```python
from build123d import *


with BuildPart() as part:
    # Sketch1 → Body (revolve)
    with BuildSketch(Plane.XY):
        with BuildLine():
            Line((0, 21), (5, 21))
            Line((5, 21), (5, 18))
            Line((5, 18), (9, 18))
            Line((9, 18), (9, 21.75))
            Line((9, 21.75), (15.9, 21.75))
            ThreePointArc((15.9, 21.75), (20.001219331, 23.448780669), (21.7, 27.55))
            Line((21.7, 27.55), (21.7, 40.25))
            Line((21.7, 40.25), (25.3, 40.25))
            Line((25.3, 40.25), (25.3, 61))
            Line((25.3, 61), (5, 61))
            Line((5, 61), (5, 66))
            Line((5, 66), (0, 66))
            Line((0, 66), (0, 21))
        make_face()
    revolve(axis=Axis((0, 0, 0), (1, 0, 0)))


solid = part.part
```
Model file for the job. Use its own axes, mm. A direction names the side the tool comes from. Coordinates: 2 decimals unless noted, no trailing zeros. Write each loop counter-clockwise with the first axis right and the second up, starting at its lowest first coordinate (ties: lowest second). Pieces come first, ordered by that corner, then holes. Notation, with made-up numbers: (-26, 67) - (20, 67) arc R9 ccw to (20, 81) - close; hole circle Ø8 at (2, 38.5). An arc over 180 degrees is marked (long way). One line per item, written item: value. Start each with the question number.
1. Tool access for faces 1 (the cylindrical face through (7.028, -2.343, 17.847)), 2 (the cylindrical face through (23.53, -40.21, 1.77)), 3 (the flat face through (5, -9, 16)): list every direction of +Z, -Z, +X, -X, +Y, -Y with a clear straight run to the whole face (end or side of a thin tool).
2. Slice it at C-C (y = 49). Write the cut outline in (x, z), plus the area to 3 significant figures.
3. Flat gauge pins, fed straight in: pin 1 (12 mm diameter, centred on x = 15, z = -22, fed in from +Y); pin 2 (13 mm diameter, centred on y = 9, z = -3, fed in from +X); pin 3 (10 mm diameter, centred on x = 19, y = 49, fed in from -Z); pin 4 (10 mm diameter, centred on x = 8.5, z = -15.5, fed in from -Y). Where does each tip first touch, or does it go through?
4. Mould opens along Z. For faces 4 (the flat face through (25.3, -40, -13)), 5 (the cylindrical face through (15.008, -48.408, -37.118)), 6 (the cylindrical face through (12.498, -2.831, 21.565)) say: released by +Z, released by -Z, zero draft, split by the parting line, or undercut.
5. Slice it at D-D (y = -42.5). Write the cut outline in (x, z), plus the area to 3 significant figures.
6. Probe line 1 (Z direction, x = 22.95, y = 0); line 2 (Z direction, x = 2.6, y = 0); line 3 (X direction, y = -27, z = 24.5). List the from-to ranges inside material, lowest first. Write a range as from..to.
7. Slice it at A-A (y = 0). Write the cut outline in (x, z), plus the area to 3 significant figures.
Answers below:
1. face 1: +X, -X
1. face 2: +X
1. face 3: -X
2. outline: (0, -44.22) - (5, -44.22) - (5, -36.33) - (25.3, -36.33) - (25.3, 36.33) - (5, 36.33) - (5, 44.22) - (0, 44.22) - close
2. area: 1,920 mm^2
3. pin 1: stops at y = 58.86
3. pin 2: passes through
3. pin 3: stops at z = -42.25
3. pin 4: stops at y = -64.91
4. face 4: zero draft
4. face 5: split by the parting line
4. face 6: undercut
5. outline: (0, -50.5) - (5, -50.5) - (5, -43.76) - (25.3, -43.76) - (25.3, 43.76) - (5, 43.76) - (5, 50.5) - (0, 50.5) - close
5. area: 2,280 mm^2
6. line 1: z = -61..-40.25, 40.25..61
6. line 2: z = -66..-21, 21..66
6. line 3: x = 0..21.7
7. outline: (0, -66) - (5, -66) - (5, -61) - (25.3, -61) - (25.3, -40.25) - (21.7, -40.25) - (21.7, -27.55) arc R5.8 ccw to (15.9, -21.75) - (9, -21.75) - (9, -18) - (5, -18) - (5, -21) - (0, -21) - close; (0, 21) - (5, 21) - (5, 18) - (9, 18) - (9, 21.75) - (15.9, 21.75) arc R5.8 ccw to (21.7, 27.55) - (21.7, 40.25) - (25.3, 40.25) - (25.3, 61) - (5, 61) - (5, 66) - (0, 66) - close
7. area: 1,930 mm^2
